Geometry check sheet. Reference: the model listing, model coordinates, mm. Give positions to 0.01 mm unless a question says otherwise; leave off trailing zeros. Loops run counter-clockwise (first coordinate to the right, second up) from the corner with the lowest first, then second, coordinate; pieces in that order, holes last.
1. Material ranges on L1, parallel to Y at x = 0, z = 1.8; L2, parallel to Z at x = 5.25, y = -9.25; L3, parallel to X at y = 1.25, z = 18.25, recorded low to high.
2. Release check for a two-part mould opening along Y. For faces 1 (the flat face through (-4, 7, 5)), 2 (the cylindrical face through (-0.867, -3.905, 10.14)), 3 (the cylindrical face through (9.692, -1.706, 2.465)), 4 (the cylindrical face through (-7.493, -0.33, 12.395)) record: +Y half, -Y half, draft (parallel to the pull), parting line (faces both ways), or undercut.
3. Cross-section at B-B, the plane y = 1. Record the cut outline in (x, z), plus the area to 3 significant figures.
4. Go/stop test with flat-tipped pins: pin 1 Ø10 at (x, z) = (-11, 17.5) entering from -Y; pin 2 Ø3.5 at (x, y) = (11, 0) entering from -Z; pin 3 Ø5 at (x, z) = (2, 16.5) entering from +Y; pin 4 Ø12 at (x, z) = (10.5, 10.5) entering from -Y. Record where each tip stops, or that it passes through.
5. Cross-section at A-A, the plane x = -1.25. Record the cut outline in (y, z), plus the area to 3 significant figures.
6. Cross-section at C-C, the plane z = 16.5. Record the cut outline in (x, y), plus the area to 3 significant figures.
7. Cross-section at D-D, the plane y = 11. Record the cut outline in (x, z), plus the area to 3 significant figures.
Autodesk Inventor part; units mm, degrees
ref_plane "YZ Plane" through (0, 0, 0) normal (1, 0, 0) x (0, 1, 0)
ref_plane "XZ Plane" through (0, 0, 0) normal (0, 1, 0) x (-1, 0, 0)
ref_plane "XY Plane" through (0, 0, 0) normal (0, 0, 1) x (1, 0, 0)
sketch "Sketch1" plane through (0, 0, 0) normal (0, 0, 1) x (1, 0, 0)
  circle A0 centre (0, 0) radius 15
  dimension "d0" = 30
extrude "Extrusion1" add sketch "Sketch1" along normal blind 5
sketch "Sketch2" plane through (0, 0, 5) normal (0, 0, 1) x (1, 0, 0)
  circle A0 centre (0, 0) radius 15
  circle A1 centre (0, 0) radius 7.5
  dimension "d4" = 15
extrude "Extrusion2" add sketch "Sketch2" along normal blind 15 contours A1
sketch "Sketch3" plane through (0, 0, 20) normal (0, 0, 1) x (1, 0, 0)
  circle A0 centre (0, 0) radius 7.5
  circle A1 centre (0, 0) radius 4
  dimension "d8" = 8
extrude "Extrusion3" cut sketch "Sketch3" against normal through all contours A1
sketch "Sketch4" plane through (0, 0, 0) normal (0, 0, -1) x (-1, 0, 0)
  circle A0 centre (0, 0) radius 4
  circle A1 centre (0, 11) radius 2.15
  dimension "d13" = 11
  dimension "d14" = 4.3
extrude "Extrusion4" cut sketch "Sketch4" against normal through all contours A1
pattern_circular "Circular Pattern1" count 4 over 360 about axis through (0, 0, 0) along (0, 0, 1) of "Extrusion4"
properties part number "lead nut"
Result:
1. L1: y = -15 to -13.15, -8.85 to -4, 4 to 8.85, 13.15 to 15
1. L2: z = 0 to 5
1. L3: x = -7.4 to -3.8, 3.8 to 7.4
2. face 1: draft
2. face 2: undercut
2. face 3: undercut
2. face 4: parting line
3. outline: (-14.97, 0) - (-12.9, 0) - (-12.9, 5) - (-14.97, 5) - close; (-9.1, 0) - (-3.87, 0) - (-3.87, 20) - (-7.43, 20) - (-7.43, 5) - (-9.1, 5) - close; (3.87, 0) - (9.1, 0) - (9.1, 5) - (7.43, 5) - (7.43, 20) - (3.87, 20) - close; (12.9, 0) - (14.97, 0) - (14.97, 5) - (12.9, 5) - close
3. area: 180 mm2
4. pin 1: stops at y = -4.5
4. pin 2: passes through
4. pin 3: stops at y = 7.5
4. pin 4: stops at y = -12.62
5. outline: (-14.95, 0) - (-12.75, 0) - (-12.75, 5) - (-14.95, 5) - close; (-9.25, 0) - (-3.8, 0) - (-3.8, 20) - (-7.4, 20) - (-7.4, 5) - (-9.25, 5) - close; (3.8, 0) - (9.25, 0) - (9.25, 5) - (7.4, 5) - (7.4, 20) - (3.8, 20) - close; (12.75, 0) - (14.95, 0) - (14.95, 5) - (12.75, 5) - close
5. area: 184 mm2
6. outline: circle Ø15 at (0, 0); hole circle Ø8 at (0, 0)
6. area: 126 mm2
7. outline: (-10.2, 0) - (-2.15, 0) - (-2.15, 5) - (-10.2, 5) - close; (2.15, 0) - (10.2, 0) - (10.2, 5) - (2.15, 5) - close
7. area: 80.5 mm2
